Autodesk Inventor part; units mm, degrees
ref_plane "YZ Plane" through (0, 0, 0) normal (1, 0, 0) x (0, 1, 0)
ref_plane "XZ Plane" through (0, 0, 0) normal (0, 1, 0) x (-1, 0, 0)
ref_plane "XY Plane" through (0, 0, 0) normal (0, 0, 1) x (1, 0, 0)
sketch "Sketch1" plane through (0, 0, 0) normal (0, 0, 1) x (1, 0, 0)
  line L0 (-76.2, -38.1) -> (76.2, -38.1)
  line L1 (76.2, -38.1) -> (76.2, 38.1)
  line L2 (76.2, 38.1) -> (-76.2, 38.1)
  line L3 (-76.2, 38.1) -> (-76.2, -38.1)
  line L4 (-76.2, -38.1) -> (76.2, 38.1) construction
  line L5 (76.2, -38.1) -> (-76.2, 38.1) construction
  point P0 (0, 0)
  dimension "d0" = 152.4
  dimension "d1" = 76.2
extrude "Extrusion1" add sketch "Sketch1" along normal blind 6.35
sketch "Sketch2" plane through (0, 0, 6.35) normal (0, 0, 1) x (1, 0, 0)
  line L0 (-177.8, -19.05) -> (25.4, -19.05)
  line L1 (25.4, -19.05) -> (25.4, 19.05)
  line L2 (25.4, 19.05) -> (-177.8, 19.05)
  line L3 (-177.8, 19.05) -> (-177.8, -19.05)
  line L4 (-76.2, 38.1) -> (-76.2, -38.1)
  line L5 (-177.8, -19.05) -> (25.4, 19.05) construction
  line L6 (25.4, -19.05) -> (-177.8, 19.05) construction
  point P0 (0, 0)
  point P1 (-76.2, 0)
  dimension "d4" = 203.2
  dimension "d5" = 38.1
extrude "Extrusion2" cut sketch "Sketch2" against normal blind 6.35
sketch "Sketch4" plane through (0, 0, 6.35) normal (0, 0, 1) x (1, 0, 0)
  point P0 (0, 0)
properties part number "Back Slide plate"
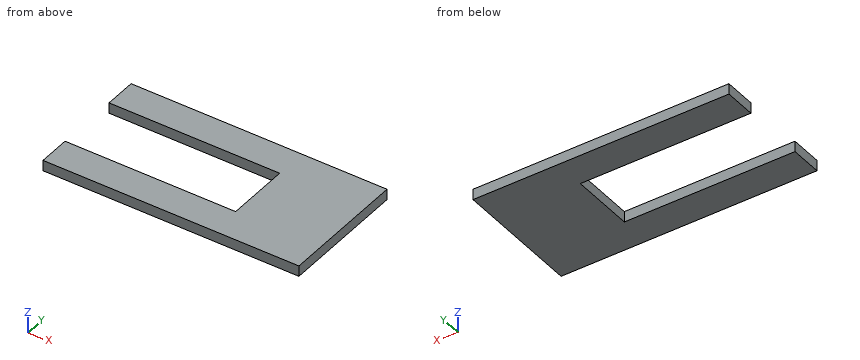
Geometry check sheet. Reference: the model listing, model coordinates, mm. Give positions to 0.01 mm unless a question says otherwise; leave off trailing zeros. Order: outer loops, then holes, each group sorted by start corner. A loop starts at its lowest first (then second) coordinate and runs counter-clockwise, first axis right, second up.
1. Section check A-A, the plane x = 2. Enter the section's corners in (y, z), and give its area (3 significant figures).
2. Section check C-C, the plane y = 5. Enter the section's corners in (x, z), and give its area (3 significant figures).
3. Thickness scan on L1, parallel to Y at x = 3.5, z = 3.75; L2, parallel to X at y = 14, z = 4.75. Record the ranges inside material, lowest first.
4. Gauge pin test, flat end, axial feed: pin 1 Ø3 at (y, z) = (0.5, 4.5) entering from -X. Record the tip position at first contact, or that the pin passes through.
5. Section check B-B, the plane z = 1.5. Enter the section's corners in (x, y).
Values follow:
1. outline: (-38.1, 0) - (-19.05, 0) - (-19.05, 6.35) - (-38.1, 6.35) - close; (19.05, 0) - (38.1, 0) - (38.1, 6.35) - (19.05, 6.35) - close
1. area: 242 mm2
2. outline: (25.4, 0) - (76.2, 0) - (76.2, 6.35) - (25.4, 6.35) - close
2. area: 323 mm2
3. L1: y = -38.1 to -19.05, 19.05 to 38.1
3. L2: x = 25.4 to 76.2
4. pin 1: stops at x = 25.4
5. outline: (-76.2, -38.1) - (76.2, -38.1) - (76.2, 38.1) - (-76.2, 38.1) - (-76.2, 19.05) - (25.4, 19.05) - (25.4, -19.05) - (-76.2, -19.05) - close
